Study the drawing (mm; zero at the part's minimum x, y, z) and answer. A direction names the side the tool comes from. Round coordinates to 2 decimals unless told otherwise and drop trailing zeros. Order: outer loops, then holes, each group sorted by start corner. A loop starts at its lowest first (then second) coordinate and runs counter-clockwise, first axis right, second up. Notation, with made-up numbers: (79, 24) -> (107, 24) arc R29 cw to (107, 54) -> close; hole circle Ø8 at (52.5, 19.25). An arc over 180 degrees is marked (long way). Use one line per item in the form item = value.
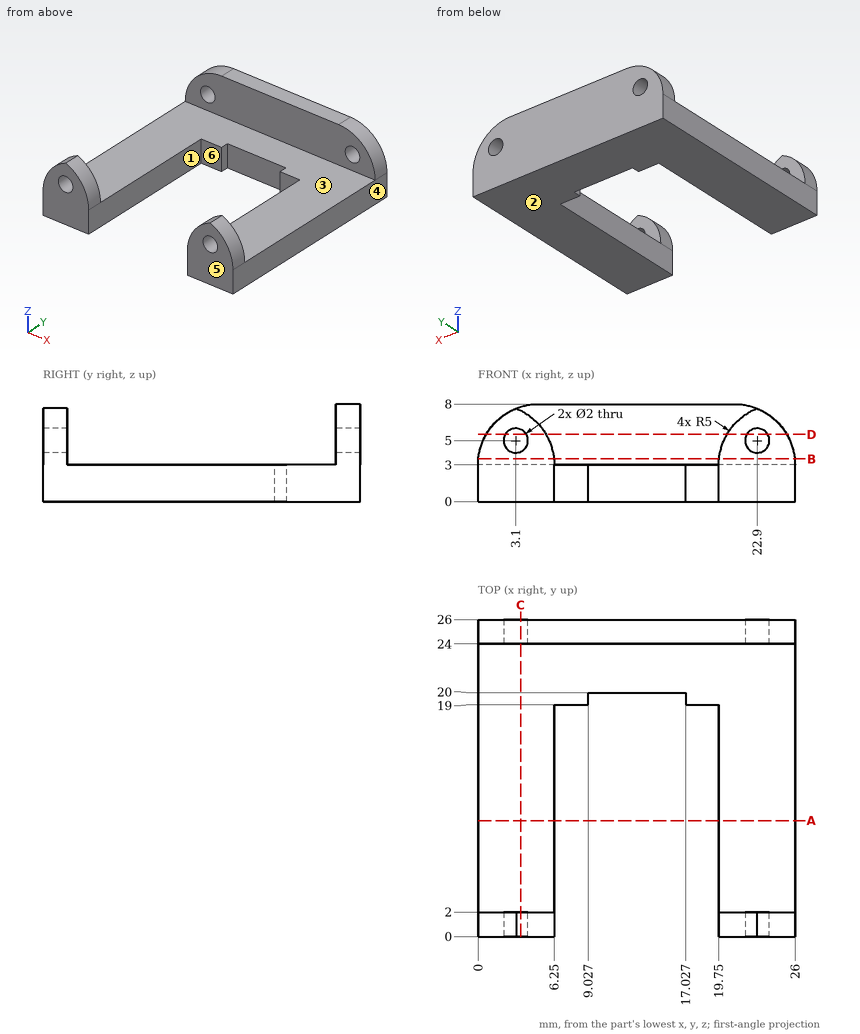
Item 1: Determine the mould class of the marked faces 4, 5 and 6 for opening direction X: released by +X, released by -X, zero draft, split by the parting line, or undercut.
Findings:
face_4 = released by +X
face_5 = zero draft
face_6 = undercut
Item 2: For the marked faces 1, 2 and 3, determine the directions among +Z, -Z, +X, -X, +Y, -Y from which every point of the face is accessible in a straight line to the end or side of a thin tool.
Findings:
face_1 = +Z, -Z, -Y
face_2 = -Z, +X, -X, +Y, -Y
face_3 = +Z, +X, -X
Item 3: The part is cut by section C-C, the plane x = 3.5. Give the vertices of the cut face in (y, z) (1 decimal).
Findings:
outline = (0, 0) -> (26, 0) -> (26, 4.1) -> (24, 4.1) -> (24, 3) -> (2, 3) -> (2, 4.1) -> (0, 4.1) -> close; (0, 5.9) -> (2, 5.9) -> (2, 7.5) -> (0, 7.5) -> close; (24, 5.9) -> (26, 5.9) -> (26, 7.8) -> (24, 7.8) -> close
Item 4: The part is cut by section B-B, the plane z = 3.5. Give the vertices of the cut face in (x, y) (1 decimal).
Findings:
outline = (0, 0) -> (6.2, 0) -> (6.2, 2) -> (0, 2) -> close; (0, 24) -> (26, 24) -> (26, 26) -> (0, 26) -> close; (19.8, 0) -> (26, 0) -> (26, 2) -> (19.8, 2) -> close
Item 5: Consider line 1 along Y through (x, z) = (1.75, 5.75); line 2 along X through (y, z) = (12, 2.75); line 3 along Y through (x, z) = (16, 2). Determine where each line is inside the solid, lowest interval first.
Findings:
line_1 = 0 to 2, 24 to 26
line_2 = 0 to 6.25, 19.75 to 26
line_3 = 20 to 26
Item 6: The part is cut by section A-A, the plane y = 9.5. Give the vertices of the cut face in (x, z).
Findings:
outline = (0, 0) -> (6.25, 0) -> (6.25, 3) -> (0, 3) -> close; (19.75, 0) -> (26, 0) -> (26, 3) -> (19.75, 3) -> close
Item 7: The part is cut by section D-D, the plane z = 5.5. Give the vertices of the cut face in (x, y).
Findings:
outline = (0.67, 0) -> (2.23, 0) -> (2.23, 2) -> (0.67, 2) -> close; (0.67, 24) -> (2.23, 24) -> (2.23, 26) -> (0.67, 26) -> close; (3.97, 0) -> (5.58, 0) -> (5.58, 2) -> (3.97, 2) -> close; (3.97, 24) -> (22.03, 24) -> (22.03, 26) -> (3.97, 26) -> close; (20.42, 0) -> (22.03, 0) -> (22.03, 2) -> (20.42, 2) -> close; (23.77, 0) -> (25.33, 0) -> (25.33, 2) -> (23.77, 2) -> close; (23.77, 24) -> (25.33, 24) -> (25.33, 26) -> (23.77, 26) -> close
Item 8: Flat-ended cylindrical pins translate along their axes: P1, Ø4, axis at x = 10.5, z = 5.5, coming from the -Y side; P2, Ø2, axis at x = 14.5, z = 1, coming from the -Y side; P3, Ø12, axis at x = 16.5, y = 15, coming from the +Z side; P4, Ø6.5, axis at x = 11.5, y = 10.5, coming from the +Z side. Find the tip coordinate at first contact, or state that the pin passes through.
Findings:
P1 = 24
P2 = 20
P3 = 3
P4 = through
